```python
from build123d import *

# Parameters (mm, degrees)
SKETCH1_W           = 80
SKETCH1_H           = 96
SKETCH1_R           = 3
BOSS_EXTRUDE1_DEPTH = 63
SKETCH2_R           = 7.5
BOSS_EXTRUDE2_DEPTH = 30


with BuildPart() as part:
    # Sketch1 → Boss-Extrude1 (new body)
    with BuildSketch(Plane(origin=(0, 0, 0), x_dir=(0, 0, -1), z_dir=(1, 0, 0))):
        with Locations((0, 8)):
            Rectangle(SKETCH1_W, SKETCH1_H)
        with Locations((0, 32)):
            Circle(SKETCH1_R, mode=Mode.SUBTRACT)
        with Locations((-32, 0)):
            Circle(SKETCH1_R, mode=Mode.SUBTRACT)
        with Locations((0, -32)):
            Circle(SKETCH1_R, mode=Mode.SUBTRACT)
        with Locations((32, 0)):
            Circle(SKETCH1_R, mode=Mode.SUBTRACT)
    extrude(amount=-BOSS_EXTRUDE1_DEPTH)

    # Sketch2 → Boss-Extrude2 (add)
    with BuildSketch(Plane(origin=(0, 0, 0), x_dir=(0, 0, -1), z_dir=(1, 0, 0))):
        Circle(SKETCH2_R)
    extrude(amount=BOSS_EXTRUDE2_DEPTH)


solid = part.part
```
Input: part model. Units: mm. Frame: model coordinates. Coordinates: 2 decimals unless noted, no trailing zeros. Write each loop counter-clockwise with the first axis right and the second up, starting at its lowest first coordinate (ties: lowest second). Pieces come first, ordered by that corner, then holes. Notation, with made-up numbers: (76, 26) - (90, 26) arc R28 cw to (90, 58) - close; hole circle Ø1 at (-12, 48.5). An arc over 180 degrees is marked (long way). Put each result on its own line as item: value. Start each with the question number.
1) Cut plane C-C (y = 0). Return the cut outline in (x, z).
2) Cut plane D-D (x = 8). Return the cut outline in (y, z).
3) Ray query, L1, parallel to Y at x = -42, z = 0; L2, parallel to Y at x = -34, z = -32; L3, parallel to X at y = 19.5, z = -16. Return the intervals inside material, ascending.
4) Contact query for flat-ended pins moving along their axis: pin 1 (5.5 mm diameter, centred on y = 32, z = 0, fed in from +X); pin 2 (12 mm diameter, centred on y = -15.5, z = 10.5, fed in from +X). Output: stop coordinate, or through.
5) Cut plane B-B (z = -32). Return the cut outline in (x, y), plus the area to 3 significant figures.
6) Cut plane A-A (y = 32). Return the cut outline in (x, z).
7) Mould query, pull axis Z, two halves, no side actions, for faces 1 (the face through (30, 0, 0)), 2 (the face through (-31, 0, 35)), 3 (the face through (14.79, 0.33, 7.493)), 4 (the face through (-31, 0, -29)). Classes: pulls with the +Z half, pulls with the -Z half, needs draft (parallel to the pull), parting line crosses it, or undercut.
Resolved:
1. outline: (-63, -40) - (0, -40) - (0, -35) - (-63, -35) - close; (-63, -29) - (0, -29) - (0, -7.5) - (30, -7.5) - (30, 7.5) - (0, 7.5) - (0, 29) - (-63, 29) - close; (-63, 35) - (0, 35) - (0, 40) - (-63, 40) - close
2. outline: circle Ø15 at (0, 0)
3. L1: y = -40 to -35, -29 to 29, 35 to 56
3. L2: y = -40 to -3, 3 to 56
3. L3: x = -63 to 0
4. pin 1: passes through
4. pin 2: stops at x = 0
5. outline: (-63, -40) - (0, -40) - (0, -3) - (-63, -3) - close; (-63, 3) - (0, 3) - (0, 56) - (-63, 56) - close
5. area: 5,670 mm2
6. outline: (-63, -40) - (0, -40) - (0, -3) - (-63, -3) - close; (-63, 3) - (0, 3) - (0, 40) - (-63, 40) - close
7. face 1: needs draft
7. face 2: undercut
7. face 3: parting line crosses it
7. face 4: undercut
